```python
from build123d import *

# Parameters (mm, degrees)
SKETCH1_R           = 8.001
SKETCH1_R_2         = 5.461
BOSS_EXTRUDE1_DEPTH = 11.461
CUT_EXTRUDE1_START  = 11.461
SKETCH1_6_R         = 5.461
CUT_EXTRUDE1_DEPTH  = 9.46


with BuildPart() as part:
    # Sketch1 → Boss-Extrude1 (new body)
    # profile 1 of 2: a face of its own
    with BuildSketch(Plane(origin=(0, 0, 0), x_dir=(1, 0, 0), z_dir=(0, 1, 0))):
        with Locations(Location((0, 0, 0), (0, 0, 90))):
            Circle(SKETCH1_R)
        Circle(SKETCH1_R_2, mode=Mode.SUBTRACT)
    # profile 2 of 2: a face of its own
    with BuildSketch(Plane(origin=(0, 0, 0), x_dir=(1, 0, 0), z_dir=(0, 1, 0))):
        Circle(SKETCH1_R_2)
    extrude(amount=BOSS_EXTRUDE1_DEPTH)

    # Sketch2 → Revolve1 (revolve)
    with BuildSketch(Plane.XY, mode=Mode.PRIVATE) as revolve1_sk:
        Polygon((0, 0), (0, -2.54), (8.001, 0), align=None)
    revolve(revolve1_sk.sketch.rotate(Axis((0, 0, 0), (0, -1, 0)), 180), axis=Axis((0, 0, 0), (0, -1, 0)))

    # Sketch1<6> → Cut-Extrude1 (cut)
    with BuildSketch(Plane(origin=(0, 0, 0), x_dir=(1, 0, 0), z_dir=(0, 1, 0)).offset(CUT_EXTRUDE1_START)):
        with Locations(Location((0, 0, 0), (0, 0, 270))):
            Circle(SKETCH1_6_R)
    extrude(amount=-CUT_EXTRUDE1_DEPTH, mode=Mode.SUBTRACT)


solid = part.part
```
Design review of the part built by this model. Coordinates are the model's own, in mm. Give positions to 0.01 mm unless a question says otherwise; leave off trailing zeros. Loops run counter-clockwise (first coordinate to the right, second up) from the corner with the lowest first, then second, coordinate; pieces in that order, holes last. Notation, with made-up numbers: M 75,-25.5 L 118,-25.5 A33 ccw 118,8.5 Z; hole C -9,-12 d7. An arc over 180 degrees is marked long. Return JSON: item names as keys, results as strings. Group by question number.
Item 1: We need section B-B (y = 0.25). Give the boundary of the cut face in (x, z).
Item 2: Insertion check: pin 1 Ø6 at (x, y) = (6, 7.5) entering from -Z; pin 2 Ø4 at (x, z) = (-6, -5) entering from -Y; pin 3 Ø6 at (x, y) = (6.5, 9) entering from -Z. Each pin has a flat end and moves straight along its axis. Give the tip position at first contact, or say it passes through.
Item 3: For probe 1 along X at (y, z) = (5.25, 0); probe 2 along Z at (x, y) = (-0.75, 4.5); probe 3 along Y at (x, z) = (1.75, -5), list the stretches that pass through material, from the lowest coordinate up.
Item 4: We need section A-A (y = 4.5). Give the boundary of the cut face in (x, z).
Item 5: Mouldability with a two-part tool opening along Z and no side actions: class faces 1 (the flat face through (5, 11.461, -3)), 2 (the flat face through (0, 2.001, 0)), 3 (the cylindrical face through (-2.092, 6.797, 5.045)), 4 (the conical face through (-0.48, -2.38, -0.15)) as released by +Z, released by -Z, zero draft, split by the parting line, or undercut.
Output:
{
 "1": {"outline": "C 0,0 d16"},
 "2": {"pin 1": "stops at z = -7.42", "pin 2": "stops at y = -0.7", "pin 3": "stops at z = -7.19"},
 "3": {"probe 1": "x = -8 to -5.46, 5.46 to 8", "probe 2": "z = -7.97 to -5.41, 5.41 to 7.97", "probe 3": "y = -0.86 to 2"},
 "4": {"outline": "C 0,0 d16; hole C 0,0 d10.92"},
 "5": {"face 1": "zero draft", "face 2": "undercut", "face 3": "undercut", "face 4": "split by the parting line"}
}
